Work out the finished part from the listing and answer in its coordinate system (mm). Round coordinates to 2 decimals unless told otherwise and drop trailing zeros. Write each loop counter-clockwise with the first axis right and the second up, starting at its lowest first coordinate (ties: lowest second). Pieces come first, ordered by that corner, then holes. Notation, with made-up numbers: (48.25, -32) - (68.25, -32) arc R23 cw to (68.25, -19) - close; hole circle Ø7 at (-20.75, 28). An arc over 180 degrees is marked (long way). Write item = value, one per line. Start each with the question number.
from build123d import *

# Parameters (mm, degrees)
SKETCH_W    = 80
SKETCH_H    = 120
SKETCH_R    = 4.5
SKETCH_R_2  = 11
SKETCH_R_3  = 3
PAD_DEPTH   = 10
FILLET_R    = 10
FILLET001_R = 1


with BuildPart() as part:
    # Sketch → Pad (new body)
    with BuildSketch(Plane.XY):
        with Locations((15, -15)):
            Rectangle(SKETCH_W, SKETCH_H)
        Circle(SKETCH_R, mode=Mode.SUBTRACT)
        with Locations((0, -30)):
            Circle(SKETCH_R_2, mode=Mode.SUBTRACT)
        with Locations((-10, -52)):
            Circle(SKETCH_R_3, mode=Mode.SUBTRACT)
        with Locations((40, -52)):
            Circle(SKETCH_R_3, mode=Mode.SUBTRACT)
        with Locations((40, 22)):
            Circle(SKETCH_R_3, mode=Mode.SUBTRACT)
        with Locations((-10, 22)):
            Circle(SKETCH_R_3, mode=Mode.SUBTRACT)
    extrude(amount=PAD_DEPTH)

    # Fillet
    fillet_edges = [part.edges().sort_by_distance(p)[0] for p in [
        (-25, -75, 5),
        (-25, 45, 5),
    ]]
    fillet(fillet_edges, radius=FILLET_R)

    # Fillet001
    fillet001_edges = [part.edges().sort_by_distance(p)[0] for p in [
        (55, -75, 5),
        (55, 45, 5),
    ]]
    fillet(fillet001_edges, radius=FILLET001_R)


solid = part.part
1. For a pull along Y with two mould halves and no side action, classify faces 1 (the face through (-22.15, 41.99, 5.07)), 2 (the face through (-25, -16, 5)), 3 (the face through (19, -75, 5)), 4 (the face through (-0.59, 4.46, 4.93)) as released by +Y, released by -Y, zero draft, split by the parting line, or undercut.
2. Find section A-A on x = 40. Give the vertices of the cut face in (y, z), plus the area to 3 significant figures.
3. Find section B-B on y = 0. Give the vertices of the cut face in (x, z), plus the area to 3 significant figures.
4. Find section D-D on y = 22. Give the vertices of the cut face in (x, z), plus the area to 3 significant figures.
5. Find section C-C on z = 3.75. Give the vertices of the cut face in (x, y), plus the area to 3 significant figures.
6. Consider line 1 (Y direction, x = 0, z = 3.5); line 2 (Y direction, x = 40, z = 5.75); line 3 (X direction, y = -51, z = 6.5). Determine where each line is inside the solid, lowest interval first.
Answer key:
q1.face_1 = released by +Y
q1.face_2 = zero draft
q1.face_3 = released by -Y
q1.face_4 = undercut
q2.outline = (-75, 0) - (-55, 0) - (-55, 10) - (-75, 10) - close; (-49, 0) - (19, 0) - (19, 10) - (-49, 10) - close; (25, 0) - (45, 0) - (45, 10) - (25, 10) - close
q2.area = 1,080 mm²
q3.outline = (-25, 0) - (-4.5, 0) - (-4.5, 10) - (-25, 10) - close; (4.5, 0) - (55, 0) - (55, 10) - (4.5, 10) - close
q3.area = 710 mm²
q4.outline = (-25, 0) - (-13, 0) - (-13, 10) - (-25, 10) - close; (-7, 0) - (37, 0) - (37, 10) - (-7, 10) - close; (43, 0) - (55, 0) - (55, 10) - (43, 10) - close
q4.area = 680 mm²
q5.outline = (-25, -65) arc R10 ccw to (-15, -75) - (54, -75) arc R1 ccw to (55, -74) - (55, 44) arc R1 ccw to (54, 45) - (-15, 45) arc R10 ccw to (-25, 35) - close; hole circle Ø6 at (-10, -52); hole circle Ø6 at (-10, 22); hole circle Ø22 at (0, -30); hole circle Ø9 at (0, 0); hole circle Ø6 at (40, -52); hole circle Ø6 at (40, 22)
q5.area = 9,000 mm²
q6.line_1 = -75 to -41, -19 to -4.5, 4.5 to 45
q6.line_2 = -75 to -55, -49 to 19, 25 to 45
q6.line_3 = -25 to -12.83, -7.17 to 37.17, 42.83 to 55
